Verification items for the finished model (mm, model axes). A direction names the side the tool comes from. Coordinates: 2 decimals unless noted, no trailing zeros. Order: outer loops, then holes, each group sorted by start corner. A loop starts at its lowest first (then second) coordinate and runs counter-clockwise, first axis right, second up.
Q1. Cross-section at A-A, the plane x = -8.5. Record the boundary of the cut face in (y, z).
Q2. Cross-section at D-D, the plane y = 2.1. Record the boundary of the cut face in (x, z).
Q3. Set-up check for faces 5 (the cylindrical face through (-10.1, 1.5, 4.1)), 6 (the flat face through (-3, 1, -10)): record each of +Z, -Z, +X, -X, +Y, -Y from which the full face is reachable in a straight line by a thin tool's end or side.
Q4. Cross-section at C-C, the plane z = 0.25. Record the boundary of the cut face in (x, y).
Q5. Cross-section at B-B, the plane x = 0. Record the boundary of the cut face in (y, z).
Q6. Draft check along X on faces 1 (the cylindrical face through (-11.4, 1.52, 9.43)), 2 (the cylindrical face through (-10.1, 1.5, -4)), 3 (the flat face through (-3, 0, 0)), 4 (the cylindrical face through (5.43, 1.52, -9.4)). Enter one of: pulls with the +X half, pulls with the -X half, needs draft (parallel to the pull), parting line crosses it, or undercut.
Q7. Thickness scan on line 1 (X direction, y = 2.5, z = -2.75); line 2 (Z direction, x = -7, y = 0.4); line 3 (X direction, y = 1.5, z = 6). Record the ranges inside material, lowest first.
from build123d import *

# Parameters (mm, degrees)
SKETCH_1_R      = 1.5
EXTRUDE_1_DEPTH = 3
FILLET_1_R      = 2


with BuildPart() as part:
    # 草图1 → 凸台-拉伸1 (new body)
    with BuildSketch(Plane(origin=(0, 0, 0), x_dir=(1, 0, 0), z_dir=(0, 1, 0))):
        Polygon((-12, -10), (-6, -10), (6, -10), (6, 10), (-6, 10), (-12, 10), align=None)
        with Locations(Location((0, -6, 0), (0, 0, 270))):
            Circle(SKETCH_1_R, mode=Mode.SUBTRACT)
        with BuildLine():
            Line((-6, -5.05), (-9.1, -5.05))
            ThreePointArc((-9.1, -5.05), (-10.1, -4.05), (-9.1, -3.05))
            Line((-9.1, -3.05), (-9.1, 3.05))
            ThreePointArc((-9.1, 3.05), (-10.1, 4.05), (-9.1, 5.05))
            Line((-9.1, 5.05), (-6, 5.05))
            ThreePointArc((-6, 5.05), (-5.292893219, 4.757106781), (-5, 4.05))
            ThreePointArc((-5, 4.05), (-5.292893219, 3.342893219), (-6, 3.05))
            Line((-6, 3.05), (-6, -3.05))
            ThreePointArc((-6, -3.05), (-5.292893219, -3.342893219), (-5, -4.05))
            ThreePointArc((-5, -4.05), (-5.292893219, -4.757106781), (-6, -5.05))
        make_face(mode=Mode.SUBTRACT)
        with Locations(Location((0, 6, 0), (0, 0, 270))):
            Circle(SKETCH_1_R, mode=Mode.SUBTRACT)
    extrude(amount=EXTRUDE_1_DEPTH)

    # 圆角1
    fillet_1_edges = [part.edges().sort_by_distance(p)[0] for p in [
        (6, 1.5, -10),
        (6, 1.5, 10),
        (-12, 1.5, 10),
        (-12, 1.5, -10),
    ]]
    fillet(fillet_1_edges, radius=FILLET_1_R)


solid = part.part
Check values:
1. outline: (0, -10) - (3, -10) - (3, -5.05) - (0, -5.05) - close; (0, 5.05) - (3, 5.05) - (3, 10) - (0, 10) - close
2. outline: (-12, -8) arc R2 ccw to (-10, -10) - (4, -10) arc R2 ccw to (6, -8) - (6, 8) arc R2 ccw to (4, 10) - (-10, 10) arc R2 ccw to (-12, 8) - close; hole (-9.1, -5.05) - (-6, -5.05) arc R1 ccw to (-6, -3.05) - (-6, 3.05) arc R1 ccw to (-6, 5.05) - (-9.1, 5.05) arc R1 ccw to (-9.1, 3.05) - (-9.1, -3.05) arc R1 ccw to start; hole circle Ø3 at (0, -6); hole circle Ø3 at (0, 6)
3. face 5: +Y, -Y
3. face 6: -Z, +X, -X, +Y, -Y
4. outline: (-12, 0) - (-9.1, 0) - (-9.1, 3) - (-12, 3) - close; (-6, 0) - (6, 0) - (6, 3) - (-6, 3) - close
5. outline: (0, -10) - (3, -10) - (3, -7.5) - (0, -7.5) - close; (0, -4.5) - (3, -4.5) - (3, 4.5) - (0, 4.5) - close; (0, 7.5) - (3, 7.5) - (3, 10) - (0, 10) - close
6. face 1: pulls with the -X half
6. face 2: undercut
6. face 3: needs draft
6. face 4: pulls with the +X half
7. line 1: x = -12 to -9.1, -6 to 6
7. line 2: z = -10 to -5.05, 5.05 to 10
7. line 3: x = -12 to -1.5, 1.5 to 6
